from build123d import *

# Parameters (mm, degrees)
F0_W     = 95.25
F0_H     = 15.875
F0_R     = 2.38125
F1_DEPTH = 3.175
F2_DEPTH = 4.7625
F3_T     = -1.5875
F4_R     = 3.175
F4_R_2   = 2.38125
F5_DEPTH = 1.5875


with BuildPart() as f1:
    # F0 (on Top) → F1 (new body)
    with BuildSketch(Plane.XY):
        Rectangle(F0_W, F0_H)
        with Locations((-43.65625, -3.96875)):
            Circle(F0_R, mode=Mode.SUBTRACT)
        with Locations((-35.71875, -3.96875)):
            Circle(F0_R, mode=Mode.SUBTRACT)
        with Locations((-27.78125, -3.96875)):
            Circle(F0_R, mode=Mode.SUBTRACT)
        with Locations((-19.84375, -3.96875)):
            Circle(F0_R, mode=Mode.SUBTRACT)
        with Locations((-11.90625, -3.96875)):
            Circle(F0_R, mode=Mode.SUBTRACT)
        with Locations((-3.96875, -3.96875)):
            Circle(F0_R, mode=Mode.SUBTRACT)
        with Locations((3.96875, -3.96875)):
            Circle(F0_R, mode=Mode.SUBTRACT)
        with Locations((11.90625, -3.96875)):
            Circle(F0_R, mode=Mode.SUBTRACT)
        with Locations((19.84375, -3.96875)):
            Circle(F0_R, mode=Mode.SUBTRACT)
        with Locations((27.78125, -3.96875)):
            Circle(F0_R, mode=Mode.SUBTRACT)
        with Locations((35.71875, -3.96875)):
            Circle(F0_R, mode=Mode.SUBTRACT)
        with Locations((43.65625, -3.96875)):
            Circle(F0_R, mode=Mode.SUBTRACT)
        with Locations((-43.65625, 3.96875)):
            Circle(F0_R, mode=Mode.SUBTRACT)
        with Locations((-35.71875, 3.96875)):
            Circle(F0_R, mode=Mode.SUBTRACT)
        with Locations((-27.78125, 3.96875)):
            Circle(F0_R, mode=Mode.SUBTRACT)
        with Locations((-19.84375, 3.96875)):
            Circle(F0_R, mode=Mode.SUBTRACT)
        with Locations((-11.90625, 3.96875)):
            Circle(F0_R, mode=Mode.SUBTRACT)
        with Locations((-3.96875, 3.96875)):
            Circle(F0_R, mode=Mode.SUBTRACT)
        with Locations((3.96875, 3.96875)):
            Circle(F0_R, mode=Mode.SUBTRACT)
        with Locations((11.90625, 3.96875)):
            Circle(F0_R, mode=Mode.SUBTRACT)
        with Locations((19.84375, 3.96875)):
            Circle(F0_R, mode=Mode.SUBTRACT)
        with Locations((27.78125, 3.96875)):
            Circle(F0_R, mode=Mode.SUBTRACT)
        with Locations((35.71875, 3.96875)):
            Circle(F0_R, mode=Mode.SUBTRACT)
        with Locations((43.65625, 3.96875)):
            Circle(F0_R, mode=Mode.SUBTRACT)
    extrude(amount=F1_DEPTH)

    # F0 (on Top) → F2 (join)
    with BuildSketch(Plane.XY):
        with Locations((-43.65625, 3.96875)):
            Circle(F0_R)
        with Locations((-43.65625, -3.96875)):
            Circle(F0_R)
        with Locations((-35.71875, -3.96875)):
            Circle(F0_R)
        with Locations((-35.71875, 3.96875)):
            Circle(F0_R)
        with Locations((-27.78125, 3.96875)):
            Circle(F0_R)
        with Locations((-19.84375, -3.96875)):
            Circle(F0_R)
        with Locations((-19.84375, 3.96875)):
            Circle(F0_R)
        with Locations((-11.90625, 3.96875)):
            Circle(F0_R)
        with Locations((-11.90625, -3.96875)):
            Circle(F0_R)
        with Locations((-27.78125, -3.96875)):
            Circle(F0_R)
        with Locations((-3.96875, -3.96875)):
            Circle(F0_R)
        with Locations((-3.96875, 3.96875)):
            Circle(F0_R)
        with Locations((3.96875, 3.96875)):
            Circle(F0_R)
        with Locations((3.96875, -3.96875)):
            Circle(F0_R)
        with Locations((11.90625, -3.96875)):
            Circle(F0_R)
        with Locations((11.90625, 3.96875)):
            Circle(F0_R)
        with Locations((19.84375, 3.96875)):
            Circle(F0_R)
        with Locations((19.84375, -3.96875)):
            Circle(F0_R)
        with Locations((27.78125, -3.96875)):
            Circle(F0_R)
        with Locations((27.78125, 3.96875)):
            Circle(F0_R)
        with Locations((35.71875, 3.96875)):
            Circle(F0_R)
        with Locations((35.71875, -3.96875)):
            Circle(F0_R)
        with Locations((43.65625, 3.96875)):
            Circle(F0_R)
        with Locations((43.65625, -3.96875)):
            Circle(F0_R)
    extrude(amount=F2_DEPTH)

    # F3
    f3_openings = [f1.faces().sort_by_distance(p)[0] for p in [
        (0, 0, 0),
    ]]
    offset(amount=F3_T, openings=f3_openings, kind=Kind.INTERSECTION)

    # F4 (on face) → F5 (join)
    with BuildSketch(Plane(origin=(0, 0, 1.5875), x_dir=(1, 0, 0), z_dir=(0, 0, -1))):
        with Locations((-39.6875, 0)):
            Circle(F4_R)
        with Locations((-39.6875, 0)):
            Circle(F4_R_2, mode=Mode.SUBTRACT)
        with Locations((-31.75, 0)):
            Circle(F4_R)
        with Locations((-31.75, 0)):
            Circle(F4_R_2, mode=Mode.SUBTRACT)
        with Locations((-23.8125, 0)):
            Circle(F4_R)
        with Locations((-23.8125, 0)):
            Circle(F4_R_2, mode=Mode.SUBTRACT)
        with Locations((-15.875, 0)):
            Circle(F4_R)
        with Locations((-15.875, 0)):
            Circle(F4_R_2, mode=Mode.SUBTRACT)
        with Locations((-7.9375, 0)):
            Circle(F4_R)
        with Locations((-7.9375, 0)):
            Circle(F4_R_2, mode=Mode.SUBTRACT)
        Circle(F4_R)
        Circle(F4_R_2, mode=Mode.SUBTRACT)
        with Locations((7.9375, 0)):
            Circle(F4_R)
        with Locations((7.9375, 0)):
            Circle(F4_R_2, mode=Mode.SUBTRACT)
        with Locations((15.875, 0)):
            Circle(F4_R)
        with Locations((15.875, 0)):
            Circle(F4_R_2, mode=Mode.SUBTRACT)
        with Locations((23.8125, 0)):
            Circle(F4_R)
        with Locations((23.8125, 0)):
            Circle(F4_R_2, mode=Mode.SUBTRACT)
        with Locations((31.75, 0)):
            Circle(F4_R)
        with Locations((31.75, 0)):
            Circle(F4_R_2, mode=Mode.SUBTRACT)
        with Locations((39.6875, 0)):
            Circle(F4_R)
        with Locations((39.6875, 0)):
            Circle(F4_R_2, mode=Mode.SUBTRACT)
    extrude(amount=F5_DEPTH)


solid = f1.part
The model under review builds one solid part; all positions refer to its coordinate system, in mm. A direction names the side the tool comes from. Coordinates: 2 decimals unless noted, no trailing zeros.
(1) Insertion check: P1, Ø4, axis at x = 0, y = 0, coming from the +Z side (3 decimals); P2, Ø0.5, axis at x = -35.5, y = -4, coming from the -Z side (3 decimals); P3, Ø5, axis at x = -40.5, y = 0, coming from the -Z side; P4, Ø2, axis at x = -43.66, y = -3.97, coming from the -Z side. Each pin has a flat end and moves straight along its axis. Give the tip position at first contact, or say it passes through.
Determined:
P1: stops at z = 3.175
P2: stops at z = 3.175
P3: stops at z = 0
P4: stops at z = 1.59
(2) Consider section B-B, the plane z = 4. Give the number of separate pieces and of enclosed holes in the cut face, plus the area to 3 significant figures.
Determined:
separate pieces: 24
enclosed holes: 0
area: 428 mm2
(3) Wall thickness on L1, parallel to Y at x = 29, z = 0.7; L2, parallel to Y at x = 20, z = 3.85; L3, parallel to Y at x = -20, z = 0.55: over which ranges is each line inside the solid? List them lowest first.
Determined:
L1: y = -7.94 to -6.35, -1.59 to 1.59, 6.35 to 7.94
L2: y = -6.34 to -1.59, 1.59 to 6.34
L3: y = -7.94 to -6.35, 6.35 to 7.94
(4) Tool access review of faces 1 (the flat face through (-32, 0, 1.588)), 2 (the cylindrical face through (-14.285, -3.864, 3.958)), 3 (the flat face through (-29, 0, 0)): name each direction out of +Z, -Z, +X, -X, +Y, -Y from which nothing blocks a thin tool from reaching the whole face with its end or side.
Determined:
face 1: -Z
face 2: +Z
face 3: -Z, +X, -X, +Y, -Y
